Check sheet for the modelled part. Datum: model origin and axes. Units: mm. A direction names the side the tool comes from. Round coordinates to 2 decimals unless told otherwise and drop trailing zeros. Write each loop counter-clockwise with the first axis right and the second up, starting at its lowest first coordinate (ties: lowest second). Pieces come first, ordered by that corner, then holes. Notation, with made-up numbers: (85, 42) -> (94, 42) arc R9 cw to (94, 52) -> close; hole circle Ø11 at (87.25, 30). An arc over 180 degrees is marked (long way). Answer as a JSON object with one key per item and string values. Group by question number.
```python
from build123d import *

# Parameters (mm, degrees)
SKETCH1_R           = 25
BOSS_EXTRUDE2_DEPTH = 750
SKETCH2_R           = 15
BOSS_EXTRUDE3_DEPTH = 70
SKETCH3_R           = 15
BOSS_EXTRUDE4_DEPTH = 35


with BuildPart() as part:
    # Sketch1 → Boss-Extrude2 (new body)
    with BuildSketch(Plane.XY):
        Circle(SKETCH1_R)
    extrude(amount=BOSS_EXTRUDE2_DEPTH)

    # Sketch2 → Boss-Extrude3 (add)
    with BuildSketch(Plane(origin=(0, 0, 0), x_dir=(-1, 0, 0), z_dir=(0, 0, -1))):
        Circle(SKETCH2_R)
    extrude(amount=BOSS_EXTRUDE3_DEPTH)

    # Sketch3 → Boss-Extrude4 (add)
    with BuildSketch(Plane.XY.offset(750)):
        Circle(SKETCH3_R)
    extrude(amount=BOSS_EXTRUDE4_DEPTH)


solid = part.part
```
(1) Section check D-D on z = 608. Record the cut outline in (x, y).
(2) Access from +Z, -Z, +X, -X, +Y, -Y to the whole of each face (thin tool, end or side, straight path). Record for faces 1 (the flat face through (11, -11, 0)), 2 (the flat face through (11, -11, 750)), 3 (the cylindrical face through (23.846, 7.509, 369.75)).
(3) Go/stop test with flat-tipped pins: pin 1 Ø5 at (x, z) = (4.5, 528) entering from +Y; pin 2 Ø4 at (x, z) = (19, 463.5) entering from +Y; pin 3 Ø1.5 at (x, z) = (-0.5, 116.5) entering from -Y. Record where each tip stops, or that it passes through.
(4) Scan lines: line 1 along Z through (x, y) = (-16, 2); line 2 along X through (y, z) = (1, 591.5); line 3 along Y through (x, z) = (-4, 24). Record each from-to range of solid material in increasing order.
(5) Section check A-A on x = 0. Record the cut outline in (y, z).
(6) Section check C-C on z = -17. Record the cut outline in (x, y), then the cut area to 3 significant figures.
Data:
{
 "1": {"outline": "circle Ø50 at (0, 0)"},
 "2": {"face 1": "-Z", "face 2": "+Z", "face 3": "+Z, -Z"},
 "3": {"pin 1": "stops at y = 24.92", "pin 2": "stops at y = 18.33", "pin 3": "stops at y = -25"},
 "4": {"line 1": "z = 0 to 750", "line 2": "x = -24.98 to 24.98", "line 3": "y = -24.68 to 24.68"},
 "5": {"outline": "(-25, 0) -> (-15, 0) -> (-15, -70) -> (15, -70) -> (15, 0) -> (25, 0) -> (25, 750) -> (15, 750) -> (15, 785) -> (-15, 785) -> (-15, 750) -> (-25, 750) -> close"},
 "6": {"outline": "circle Ø30 at (0, 0)", "area": "707 mm²"}
}
